CAD build for the part. Positions are in the model's coordinates, mm. A direction names the side the tool comes from. Coordinates: 2 decimals unless noted, no trailing zeros. Order: outer loops, then holes, each group sorted by start corner. A loop starts at its lowest first (then second) coordinate and runs counter-clockwise, first axis right, second up.
Autodesk Inventor part; units mm, degrees
ref_plane "YZ Plane" through (0, 0, 0) normal (1, 0, 0) x (0, 1, 0)
ref_plane "XZ Plane" through (0, 0, 0) normal (0, 1, 0) x (-1, 0, 0)
ref_plane "XY Plane" through (0, 0, 0) normal (0, 0, 1) x (1, 0, 0)
sketch "Sketch_1" plane through (0, 0, 0) normal (0, 0, 1) x (1, 0, 0)
  line L0 (5, 0) -> (-7, 0)
  line L1 (-7, 0) -> (-7, 4)
  line L2 (-7, 4) -> (-5, 4)
  line L3 (-5, 4) -> (-5, 2.5)
  line L4 (-5, 2.5) -> (0, 2.5)
  line L5 (0, 2.5) -> (0, 1.5)
  line L6 (0, 1.5) -> (4.6935, 1.5)
  line L7 (4.6935, 1.5) -> (5, 1.1935)
  line L8 (5, 1.1935) -> (5, 0)
  line L9 (5, 0) -> (-7, 0)
revolve "Revolution1" add sketch "Sketch_1" angle 360 about axis through (5, 0, 0) along (1, 0, 0)
thread "Thread1"
sketch "Sketch_2" plane through (-7, 0, 0) normal (-1, 0, 0) x (0, 1, 0)
  line L0 (-1.1547, 0) -> (-0.5774, -1)
  line L1 (-0.5774, -1) -> (0.5774, -1)
  line L2 (0.5774, -1) -> (1.1547, 0)
  line L3 (1.1547, 0) -> (0.5774, 1)
  line L4 (0.5774, 1) -> (-0.5774, 1)
  line L5 (-0.5774, 1) -> (-1.1547, 0)
extrude "Extrusion1" cut sketch "Sketch_2" against normal blind 2
sketch "Sketch_3" plane through (0, 0, 0) normal (0, 0, 1) x (1, 0, 0)
  line L0 (-4.4226, 0) -> (-5, 0)
  line L1 (-5, 0) -> (-5, 1)
  line L2 (-5, 1) -> (-4.4226, 0)
  line L3 (-4.4226, 0) -> (-5, 0)
revolve "Revolution2" cut sketch "Sketch_3" angle 360 about axis through (-4.4226, 0, 0) along (1, 0, 0)
properties part number "DBB3-5-5"
1) Slice it at A-A (x = -3.25). List the corners of the cut face in (y, z), plus the area to 3 significant figures.
2) Slice it at C-C (y = 1.75). List the corners of the cut face in (x, z), plus the area to 3 significant figures.
3) Two-plate mould, pull along Y, no slides. Class faces 1 (the flat face through (-6.01, 0.86, 0.51)), 2 (the flat face through (-6, 0, 1)), 3 (the flat face through (0, 2, 0)), 4 (the cylindrical face through (-5.986, -0.867, -3.905)): released by +Y, released by -Y, zero draft, split by the parting line, or undercut.
4) Drill centre lines: probe 1 along X at (y, z) = (2, -0.5); probe 2 along X at (y, z) = (1, 3.75); probe 3 along Y at (x, z) = (0.5, -0.25). Where is each one in solid material? Low to high.
5) Which spindle directions (+Z, -Z, +X, -X, +Y, -Y) get a long thin tool onto all of the face, cutting with end or side? Do faces 5 (the cylindrical face through (-2.46, -0.54, -2.44)), 6 (the flat face through (-6.01, 0.87, -0.49)), 7 (the flat face through (5, 0, 0)). Say none if no direction does.
6) Slice it at D-D (x = 2.5). List the corners of the cut face in (y, z).
7) Pin check, flat tips, straight feed: P1, Ø1.5, axis at x = 3, z = 2.5, coming from the +Y side; P2, Ø0.9, axis at y = 0.5, z = 0.5, coming from the -X side; P3, Ø1.5, axis at x = -5, z = -2, coming from the +Y side; P4, Ø1.5, axis at x = 3.5, z = 0, coming from the +Y side. Stop position of each tip, or through.
8) Slice it at B-B (z = 2.25). List the corners of the cut face in (x, y), plus the area to 3 significant figures.
Worked out:
1. outline: circle Ø5 at (0, 0)
1. area: 19.6 mm2
2. outline: (-7, -3.6) - (-5, -3.6) - (-5, -1.79) - (0, -1.79) - (0, 1.79) - (-5, 1.79) - (-5, 3.6) - (-7, 3.6) - close
2. area: 32.2 mm2
3. face 1: undercut
3. face 2: undercut
3. face 3: zero draft
3. face 4: split by the parting line
4. probe 1: x = -7 to 0
4. probe 2: x = -7 to -5
4. probe 3: y = -1.48 to 1.48
5. face 5: +X
5. face 6: -X
5. face 7: +Z, -Z, +X, +Y, -Y
6. outline: circle Ø3 at (0, 0)
7. P1: passes through
7. P2: stops at x = -7
7. P3: stops at y = 3.8
7. P4: stops at y = 1.5
8. outline: (-7, -3.31) - (-5, -3.31) - (-5, -1.09) - (0, -1.09) - (0, 1.09) - (-5, 1.09) - (-5, 3.31) - (-7, 3.31) - close
8. area: 24.1 mm2
